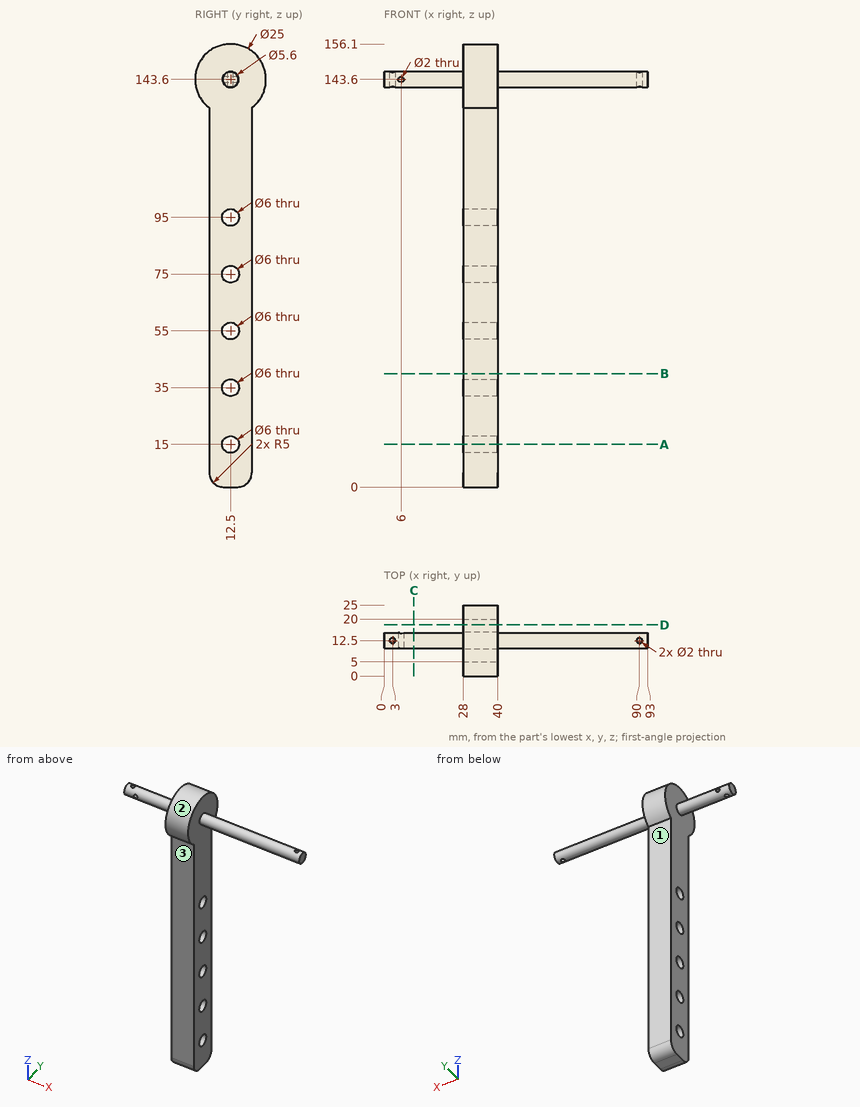
Answer from the drawing. Dimensions are ordinates in mm from the lowest x, y and z of the part. A direction names the side the tool comes from. Coordinates: 2 decimals unless noted, no trailing zeros. Write each loop counter-clockwise with the first axis right and the second up, starting at its lowest first coordinate (ties: lowest second). Pieces come first, ordered by that corner, then holes. Notation, with made-up numbers: (-39.75, 48) - (-6.75, 48) arc R15 ccw to (-6.75, 67) - close; hole circle Ø10 at (32.25, 31.5). An arc over 180 degrees is marked (long way). Answer as CSV lines item,"result".
1. A tool of negligible diameter and unlimited length cuts with its end or side. For the marked faces 1, 2 and 3, from which of +Z, -Z, +X, -X, +Y, -Y can it reach the whole face along a straight path? Write none if from no direction.
Computed values:
face 1,"-Z, +X, -X, +Y"
face 2,"+X, -X"
face 3,"-Z, +X, -X, -Y"
2. Find section A-A (z = 15). Give the vertices of the cut face in (x, y).
Computed values:
outline,"(28, 5) - (40, 5) - (40, 9.5) - (28, 9.5) - close; (28, 15.5) - (40, 15.5) - (40, 20) - (28, 20) - close"
3. Given P1, Ø3.5, axis at x = 35.5, z = 83, coming from the +Y side; P2, Ø7.5, axis at y = 16, z = 78.5, coming from the +X side; P3, Ø12, axis at x = 45.5, z = 118.5, coming from the -Y side, each flat-ended and moving along its own axis, determine where each tip first touches the part or whether it passes through.
Computed values:
P1,"stops at y = 20"
P2,"stops at x = 40"
P3,"stops at y = 5"
4. Find section C-C (x = 10.5). Give the vertices of the cut face in (y, z), plus the area to 3 significant figures.
Computed values:
outline,"circle Ø5.6 at (12.5, 143.6)"
area,"24.6 mm²"
5. Find section D-D (y = 18). Give the vertices of the cut face in (x, z).
Computed values:
outline,"(28, 1) - (40, 1) - (40, 154.82) - (28, 154.82) - close"
6. Straight lines are drawn through the part: line 1 (X direction, y = 12.55, z = 143.6); line 2 (Y direction, x = 37, z = 75); line 3 (X direction, y = 11.75, z = 58). For each, find the intervals that lie inside material, in ascending order. Write a range as [from, to].
Computed values:
line 1,"x = [0, 2], [4, 5], [7, 89], [91, 93]"
line 2,"y = [5, 9.5], [15.5, 20]"
line 3,"x = [28, 40]"
7. Find section B-B (z = 40). Give the vertices of the cut face in (x, y), plus the area to 3 significant figures.
Computed values:
outline,"(28, 5) - (40, 5) - (40, 20) - (28, 20) - close"
area,"180 mm²"
